Job drawing, mm, ordinate dimensions from the low corner. One solid piece. Coordinates: 2 decimals unless noted, no trailing zeros. Order: outer loops, then holes, each group sorted by start corner. A loop starts at its lowest first (then second) coordinate and runs counter-clockwise, first axis right, second up. Notation, with made-up numbers: M -24.75,-23.5 L 8.25,-23.5 A27 ccw 8.25,15.5 Z; hole C 81.5,57 d1. An arc over 180 degrees is marked long. Write item = value, one per line.
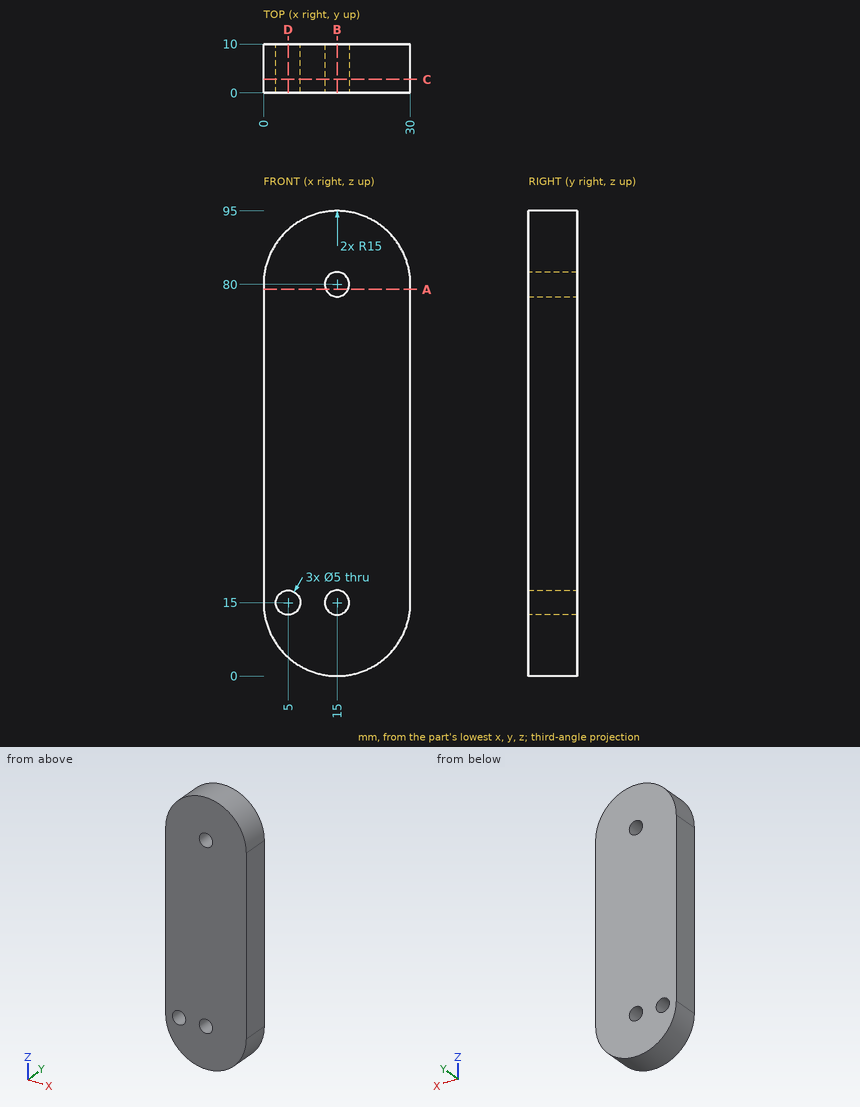
(1) Slice it at A-A, the plane z = 79. Write the cut outline in (x, y), then the cut area to 3 significant figures.
Evaluation:
outline = M 0,0 L 12.71,0 L 12.71,10 L 0,10 Z; M 17.29,0 L 30,0 L 30,10 L 17.29,10 Z
area = 254 mm²
(2) Slice it at C-C, the plane y = 2.75. Write the cut outline in (x, z), then the cut area to 3 significant figures.
Evaluation:
outline = M 0,15 A15 ccw 30,15 L 30,80 A15 ccw 0,80 Z; hole C 5,15 d5; hole C 15,15 d5; hole C 15,80 d5
area = 2,600 mm²
(3) Pin check, flat tips, straight feed: pin 1 Ø3 at (x, z) = (15, 15) entering from +Y; pin 2 Ø6 at (x, y) = (23.5, 7) entering from -Z. Stop position of each tip, or through.
Evaluation:
pin_1 = through
pin_2 = 1.04
(4) Slice it at D-D, the plane x = 5. Write the cut outline in (y, z).
Evaluation:
outline = M 0,3.82 L 10,3.82 L 10,12.5 L 0,12.5 Z; M 0,17.5 L 10,17.5 L 10,91.18 L 0,91.18 Z
(5) Slice it at B-B, the plane x = 15. Write the cut outline in (y, z).
Evaluation:
outline = M 0,0 L 10,0 L 10,12.5 L 0,12.5 Z; M 0,17.5 L 10,17.5 L 10,77.5 L 0,77.5 Z; M 0,82.5 L 10,82.5 L 10,95 L 0,95 Z
(6) Wall check: line 1 (X direction, y = 4.75, z = 15); line 2 (Z direction, x = 14.75, y = 4); line 3 (Z direction, x = 13, y = 3.75). Give the ranges that are in metal, low to high. Write a range as from..to.
Evaluation:
line_1 = 0..2.5, 7.5..12.5, 17.5..30
line_2 = 0..12.51, 17.49..77.51, 82.49..95
line_3 = 0.13..13.5, 16.5..78.5, 81.5..94.87
